The drawing under review shows one solid part. Ordinate dimensions are in mm from its lowest x, y, z. Round coordinates to 2 decimals unless told otherwise and drop trailing zeros. Write each loop counter-clockwise with the first axis right and the second up, starting at its lowest first coordinate (ties: lowest second). Pieces come first, ordered by that corner, then holes. Notation, with made-up numbers: M 71,17.5 L 100,17.5 A27 ccw 100,41.5 Z; hole C -13,45 d1. An arc over 180 degrees is marked long. One line per item, written item: value. Start each with the question number.
1) Take a section at C-C, the plane y = 35. Write out the cut boundary in (x, z) (1 decimal), and give its area (3 significant figures).
2) For P1, Ø1.6, axis at y = 39.5, z = 2, coming from the +X side; P2, Ø1.6, axis at y = 52.5, z = 1, coming from the -X side, all flat-tipped, find the tip position at first contact; note any pin that passes through.
3) Wall thickness on probe 1 along X at (y, z) = (12.5, 1.65); probe 2 along Y at (x, z) = (45, 1.85); probe 3 along X at (y, z) = (43.5, 2.3): over which ranges is each line inside the solid? List them lowest first.
4) Take a section at B-B, the plane x = 28. Write out the cut boundary in (y, z) (1 decimal).
5) Take a section at A-A, the plane z = 1.5. State how many separate pieces and enclosed holes the cut face has.
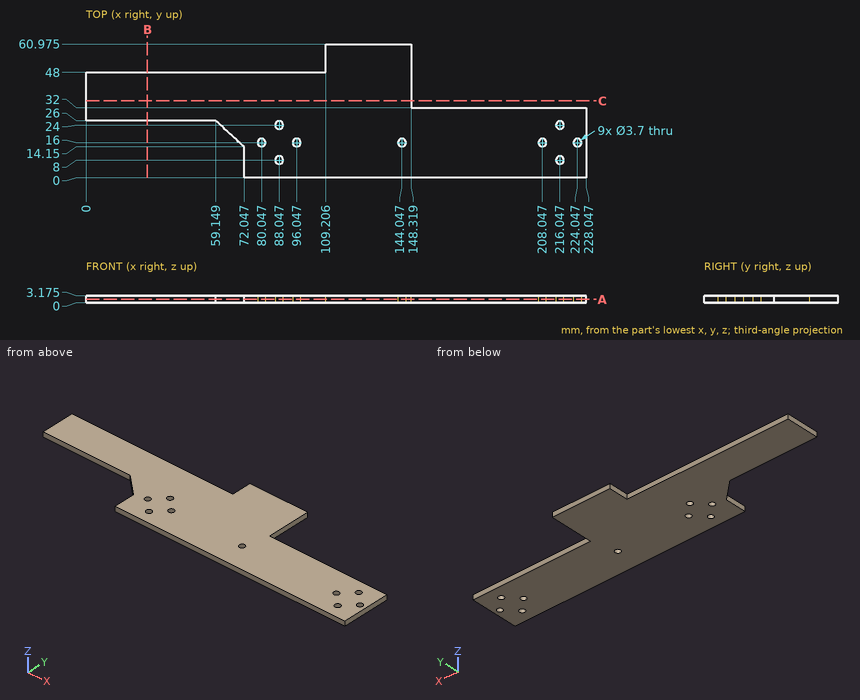
Checked values:
1. outline: M 0,0 L 148.3,0 L 148.3,3.2 L 0,3.2 Z
1. area: 471 mm2
2. P1: stops at x = 148.32
2. P2: stops at x = 109.21
3. probe 1: x = 72.05 to 228.05
3. probe 2: y = 26 to 48
3. probe 3: x = 0 to 148.32
4. outline: M 26,0 L 48,0 L 48,3.2 L 26,3.2 Z
5. separate pieces: 1
5. enclosed holes: 9
